Check sheet for the modelled part. Datum: model origin and axes. Units: mm. Round coordinates to 2 decimals unless told otherwise and drop trailing zeros. Loops run counter-clockwise (first coordinate to the right, second up) from the corner with the lowest first, then second, coordinate; pieces in that order, holes last. Notation, with made-up numbers: (-33, -6.75) - (-29, -6.75) arc R18 cw to (-29, 24.25) - close; hole circle Ø5 at (-5, 35). An arc over 180 degrees is marked (long way). Answer in a Markdown table with one row per item. Add a question column.
(1) Cross-section at A-A on y = 3. Enter the section's corners in (x, z), then the cut area to 3 significant figures.
(2) Cross-section at B-B on x = 10. Enter the section's corners in (y, z).
(3) Thickness scan on line 1 along X through (y, z) = (1, 9); line 2 along X through (y, z) = (14, 7.75); line 3 along Z through (x, y) = (10, 8.5). Record the ranges inside material, lowest first.
(4) Gauge pin test, flat end, axial feed: pin 1 (1.8 mm diameter, centred on x = 0, z = 9, fed in from +Y). Record the tip position at first contact, or that the pin passes through.
from build123d import *

# Parameters (mm, degrees)
F0_W     = 50
F0_H     = 50
F1_DEPTH = 10
F3_DEPTH = 50.001


# Not quite as in the source:
# - a feature names something its author has since deleted; it is built from what else it names


with BuildPart() as f1:
    # F0 (on Top) → F1 (new body)
    with BuildSketch(Plane.XY):
        Rectangle(F0_W, F0_H)
    extrude(amount=F1_DEPTH)

    # F2 (on face) → F3 (cut, through all)
    with BuildSketch(Plane.XZ.offset(25)):
        with BuildLine():
            Line((8.8819660113, 10), (11.1180339887, 10))
            ThreePointArc((11.1180339887, 10), (10, 10.5), (8.8819660113, 10))
        make_face()
        with BuildLine():
            ThreePointArc((1.1180339887, 10), (0, 10.5), (-1.1180339887, 10))
            Line((-1.1180339887, 10), (1.1180339887, 10))
        make_face()
        with BuildLine():
            ThreePointArc((-8.8819660113, 10), (-10, 10.5), (-11.1180339887, 10))
            Line((-11.1180339887, 10), (-8.8819660113, 10))
        make_face()
        with BuildLine():
            ThreePointArc((-18.8819660113, 10), (-20, 10.5), (-21.1180339887, 10))
            Line((-21.1180339887, 10), (-18.8819660113, 10))
        make_face()
        with BuildLine():
            ThreePointArc((11.5, 9), (11.4012585384, 9.5352331347), (11.1180339887, 10))
            Line((11.1180339887, 10), (8.8819660113, 10))
            ThreePointArc((8.8819660113, 10), (9.4647668653, 7.5987414616), (11.5, 9))
        make_face()
        with BuildLine():
            Line((1.1180339887, 10), (-1.1180339887, 10))
            ThreePointArc((-1.1180339887, 10), (-0.5352331347, 7.5987414616), (1.5, 9))
            ThreePointArc((1.5, 9), (1.4012585384, 9.5352331347), (1.1180339887, 10))
        make_face()
        with BuildLine():
            Line((-8.8819660113, 10), (-11.1180339887, 10))
            ThreePointArc((-11.1180339887, 10), (-10.5352331347, 7.5987414616), (-8.5, 9))
            ThreePointArc((-8.5, 9), (-8.5987414616, 9.5352331347), (-8.8819660113, 10))
        make_face()
        with BuildLine():
            Line((-18.8819660113, 10), (-21.1180339887, 10))
            ThreePointArc((-21.1180339887, 10), (-20.5352331347, 7.5987414616), (-18.5, 9))
            ThreePointArc((-18.5, 9), (-18.5987414616, 9.5352331347), (-18.8819660113, 10))
        make_face()
        with BuildLine():
            ThreePointArc((21.5, 9), (21.4012585384, 9.5352331347), (21.1180339887, 10))
            Line((21.1180339887, 10), (18.8819660113, 10))
            ThreePointArc((18.8819660113, 10), (19.4647668653, 7.5987414616), (21.5, 9))
        make_face()
    extrude(amount=-F3_DEPTH, mode=Mode.SUBTRACT)


solid = f1.part
Answers:
| question | item | result |
|---|---|---|
| 1 | outline | (-25, 0) - (25, 0) - (25, 10) - (21.12, 10) arc R1.5 cw (long way) to (18.88, 10) - (11.12, 10) arc R1.5 cw (long way) to (8.88, 10) - (1.12, 10) arc R1.5 cw (long way) to (-1.12, 10) - (-8.88, 10) arc R1.5 cw (long way) to (-11.12, 10) - (-18.88, 10) arc R1.5 cw (long way) to (-21.12, 10) - (-25, 10) - close |
| 1 | area | 469 mm^2 |
| 2 | outline | (-25, 0) - (25, 0) - (25, 7.5) - (-25, 7.5) - close |
| 3 | line 1 | x = -25 to -21.5, -18.5 to -11.5, -8.5 to -1.5, 1.5 to 8.5, 11.5 to 18.5, 21.5 to 25 |
| 3 | line 2 | x = -25 to -20.83, -19.17 to -10.83, -9.17 to -0.83, 0.83 to 9.17, 10.83 to 19.17, 20.83 to 25 |
| 3 | line 3 | z = 0 to 7.5 |
| 4 | pin 1 | passes through |
